from build123d import *

# Parameters (mm, degrees)
SALIENTE_EXTRUIR2_DEPTH    = 55
CROQUIS6_R                 = 21.05
CORTAR_EXTRUIR1_DEPTH      = 7
CORTAR_EXTRUIR2_DEPTH      = 73.286420098
CORTAR_EXTRUIR2_DEPTH_BACK = 73.286420098
CROQUIS8_R                 = 15
CORTAR_EXTRUIR3_DEPTH      = 72.703044082
CORTAR_EXTRUIR3_DEPTH_BACK = 72.703044082
CROQUIS9_R                 = 1.6
CHAFL_N1_SIZE              = 5
CROQUIS11_W                = 10
CROQUIS11_H                = 5
SALIENTE_EXTRUIR3_DEPTH    = 20
CROQUIS12_W                = 10
CROQUIS12_H                = 3
SALIENTE_EXTRUIR4_DEPTH    = 9
CROQUIS13_W                = 10
CROQUIS13_H                = 5
SALIENTE_EXTRUIR5_DEPTH    = 20


with BuildPart() as part:
    # Croquis4 → Saliente-Extruir2 (new body)
    with BuildSketch(Plane.XY):
        Polygon((-31.428571429, 5.761904762), (-31.428571429, 14.761904762), (-41.428571429, 14.761904762), (-41.428571429, 19.761904762), (-26.428571429, 19.761904762), (-26.428571429, 4.761904762), (28.571428571, 4.761904762), (28.571428571, -5.238095238), (-31.428571429, -5.238095238), align=None)
    extrude(amount=SALIENTE_EXTRUIR2_DEPTH)

    # Croquis6 → Cortar-Extruir1 (cut)
    with BuildSketch(Plane(origin=(0, 4.761904762, 0), x_dir=(1, 0, 0), z_dir=(0, 1, 0))):
        with Locations(Location((3.571428571, -27.5, 0), (0, 0, 180))):
            Circle(CROQUIS6_R)
    extrude(amount=-CORTAR_EXTRUIR1_DEPTH, mode=Mode.SUBTRACT)

    # Croquis8 → Cortar-Extruir2 (cut, two sides: drawn at the far end of the back side and taken through both)
    with BuildSketch(Plane(origin=(0, -2.238095238, 0), x_dir=(1, 0, 0), z_dir=(0, 1, 0)).offset(-CORTAR_EXTRUIR2_DEPTH_BACK)):
        with Locations(Location((3.571428571, -27.5, 0), (0, 0, 180))):
            Circle(CROQUIS8_R)
    extrude(amount=CORTAR_EXTRUIR2_DEPTH + CORTAR_EXTRUIR2_DEPTH_BACK, mode=Mode.SUBTRACT)

    # Croquis9 → Cortar-Extruir3 (cut, two sides: drawn at the far end of the back side and taken through both)
    with BuildSketch(Plane.XZ.offset(-14.761904762).offset(-CORTAR_EXTRUIR3_DEPTH_BACK)):
        with Locations((-36.428571429, 45.5)):
            Circle(CROQUIS9_R)
        with Locations(Location((-36.428571429, 9.5, 0), (0, 0, 180))):
            Circle(CROQUIS9_R)
    extrude(amount=CORTAR_EXTRUIR3_DEPTH + CORTAR_EXTRUIR3_DEPTH_BACK, mode=Mode.SUBTRACT)

    # Chaflán1
    chafl_n1_edges = [part.edges().sort_by_distance(p)[0] for p in [
        (-31.428571429, -5.238095238, 27.5),
        (-26.428571429, 4.761904762, 27.5),
    ]]
    chamfer(chafl_n1_edges, length=CHAFL_N1_SIZE)

    # Croquis11 → Saliente-Extruir3 (add)
    with BuildSketch(Plane(origin=(0, 4.761904762, 0), x_dir=(1, 0, 0), z_dir=(0, 1, 0))):
        with Locations((18.571428571, -52.5)):
            Rectangle(CROQUIS11_W, CROQUIS11_H)
    extrude(amount=SALIENTE_EXTRUIR3_DEPTH)

    # Croquis12 → Saliente-Extruir4 (add)
    with BuildSketch(Plane.XY.offset(55)):
        with Locations((18.571428571, 23.261904762)):
            Rectangle(CROQUIS12_W, CROQUIS12_H)
    extrude(amount=SALIENTE_EXTRUIR4_DEPTH)

    # Croquis13 → Saliente-Extruir5 (add)
    with BuildSketch(Plane(origin=(0, 4.761904762, 0), x_dir=(1, 0, 0), z_dir=(0, 1, 0))):
        with Locations((20.071428571, -5.5)):
            Rectangle(CROQUIS13_W, CROQUIS13_H)
    extrude(amount=SALIENTE_EXTRUIR5_DEPTH)


solid = part.part
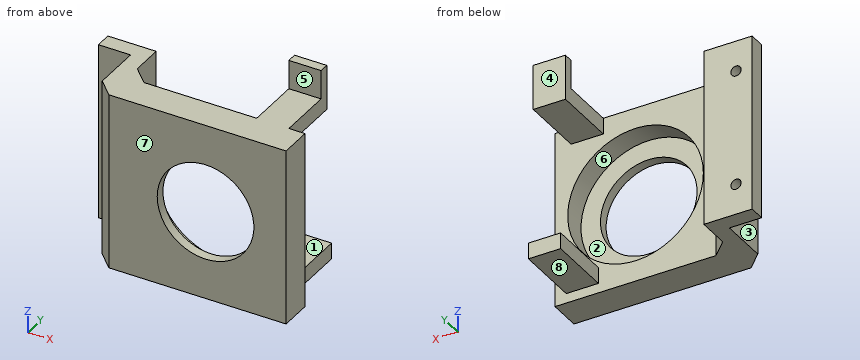
Geometry check sheet. Reference: the model listing, model coordinates, mm. Face numbers are marked on the shaded views. A direction names the side the tool comes from. Round coordinates to 2 decimals unless told otherwise and drop trailing zeros. Loops run counter-clockwise (first coordinate to the right, second up) from the corner with the lowest first, then second, coordinate; pieces in that order, holes last. Notation, with made-up numbers: (-15.5, 81.5) - (11.5, 81.5) arc R13 ccw to (11.5, 93.5) - close; hole circle Ø1 at (35.25, -18.75). An arc over 180 degrees is marked (long way). One line per question, with ' | ' between items. Start each with the question number.
1. Draft check along Z on the marked faces 6, 7 and 8. Enter one of: released by +Z, released by -Z, zero draft, split by the parting line, or undercut.
2. Scan lines: line 1 (X direction, y = 16, z = 7); line 2 (Z direction, x = 23.5, y = 23.5); line 3 (X direction, y = 18.25, z = 29). Record each from-to range of solid material in increasing order. Write a range as [from, to].
3. Cross-section at A-A on z = 27.5. Record the cut outline in (x, y), then the cut area to 3 significant figures.
4. Tool access check on the marked faces 1, 2, 3, 4 and 5. Record the directions out of +Z, -Z, +X, -X, +Y, -Y that give a thin tool (end or side, any length) a straight path to the whole face; none if there is none.
5. Depth check by flat-ended pin: pin 1 (2 mm diameter, centred on x = -33, y = 1.5, fed in from +Z); pin 2 (1.5 mm diameter, centred on x = 18, z = 21.5, fed in from +Y); pin 3 (1 mm diameter, centred on x = 2.5, y = 1.5, fed in from +Z); pin 4 (4.5 mm diameter, centred on x = 19.5, z = 59, fed in from -Y). Enter the tip coordinate at first touch or a pass-through.
6. Cross-section at C-C on x = -15. Record the cut outline in (y, z).
7. Cross-section at D-D on z = 45.5. Record the cut outline in (x, y).
8. Cross-section at B-B on y = 22.75. Record the cut outline in (x, z).
Taken from the geometry:
1) face 6: undercut | face 7: zero draft | face 8: released by -Z
2) line 1: [-41.43, -26.43], [15.07, 25.07] | line 2: [3, 8], [50, 64] | line 3: [-41.43, -26.43]
3) outline: (-41.43, 14.76) - (-31.43, 14.76) - (-31.43, -0.24) - (-26.43, -5.24) - (-11.43, -5.24) - (-11.43, -2.24) - (-17.48, -2.24) - (-17.48, 4.76) - (-21.43, 4.76) - (-26.43, 9.76) - (-26.43, 19.76) - (-41.43, 19.76) - close; (18.57, -5.24) - (28.57, -5.24) - (28.57, 4.76) - (24.62, 4.76) - (24.62, -2.24) - (18.57, -2.24) - close | area: 340 mm²
4) face 1: +X, +Y | face 2: +Y | face 3: +Z, -Z, -X, -Y | face 4: +Z, -Z, +X, -X, +Y | face 5: +Z, +X, -X, -Y
5) pin 1: through | pin 2: y = -2.24 | pin 3: z = 55 | pin 4: y = 21.76
6) outline: (-5.24, 0) - (4.76, 0) - (4.76, 17.59) - (-2.24, 17.59) - (-2.24, 37.41) - (4.76, 37.41) - (4.76, 55) - (-5.24, 55) - close
7) outline: (-41.43, 14.76) - (-38.03, 14.76) - (-38.03, 19.76) - (-41.43, 19.76) - close; (-34.83, 14.76) - (-31.43, 14.76) - (-31.43, -0.24) - (-26.43, -5.24) - (28.57, -5.24) - (28.57, 4.76) - (14.48, 4.76) - (14.48, -2.24) - (-7.34, -2.24) - (-7.34, 4.76) - (-21.43, 4.76) - (-26.43, 9.76) - (-26.43, 19.76) - (-34.83, 19.76) - close
8) outline: (13.57, 50) - (23.57, 50) - (23.57, 64) - (13.57, 64) - close; (15.07, 3) - (25.07, 3) - (25.07, 8) - (15.07, 8) - close
